from build123d import *

# Parameters (mm, degrees)
CROQUIS1_W              = 12
CROQUIS1_H              = 10
CROQUIS1_R              = 0.5
SALIENTE_EXTRUIR1_DEPTH = 0.7
CROQUIS2_R              = 1.5
SALIENTE_EXTRUIR2_DEPTH = 8.3
SALIENTE_EXTRUIR3_DEPTH = 0.7
SALIENTE_EXTRUIR4_DEPTH = 0.7
CORTAR_EXTRUIR1_REACH   = 13.916
CROQUIS5_R              = 1.5
REDONDEO1_R             = 0.5


with BuildPart() as part:
    # Croquis1 → Saliente-Extruir1 (new body)
    with BuildSketch(Plane(origin=(0, 0, 0), x_dir=(1, 0, 0), z_dir=(0, 1, 0))):
        Rectangle(CROQUIS1_W, CROQUIS1_H)
        with Locations(Location((0, 0, 0), (0, 0, 270))):
            Circle(CROQUIS1_R, mode=Mode.SUBTRACT)
    extrude(amount=SALIENTE_EXTRUIR1_DEPTH)

    # Croquis2 → Saliente-Extruir2 (add)
    with BuildSketch(Plane(origin=(0, 0.7, 0), x_dir=(1, 0, 0), z_dir=(0, 1, 0))):
        with Locations(Location((4, 3, 0), (0, 0, 90))):
            Circle(CROQUIS2_R)
        with Locations(Location((-4, -3, 0), (0, 0, 90))):
            Circle(CROQUIS2_R)
    extrude(amount=SALIENTE_EXTRUIR2_DEPTH)

    # Croquis3 → Saliente-Extruir3 (add)
    with BuildSketch(Plane(origin=(0, 3.3, 0), x_dir=(1, 0, 0), z_dir=(0, 1, 0))):
        Polygon((6, -0.6), (1.6, -0.6), (1.6, -5), (-6, -5), (-6, 5), (6, 5), align=None)
    extrude(amount=SALIENTE_EXTRUIR3_DEPTH)

    # Croquis4 → Saliente-Extruir4 (add)
    with BuildSketch(Plane(origin=(0, 8.3, 0), x_dir=(1, 0, 0), z_dir=(0, 1, 0))):
        Polygon((6, -0.6), (6, -5), (1.6, -5), (-6, -5), (-6, 5), (6, 5), align=None)
    extrude(amount=SALIENTE_EXTRUIR4_DEPTH)

    # Cortar-Extruir1: up to this face of the body (flat: up to its plane)
    cortar_extruir1_end = Plane(part.part.faces().sort_by_distance((-0.850469255, 3.3, -0.626661556))[0])
    # Croquis5 → Cortar-Extruir1 (cut, up to the picked face)
    with BuildSketch(Plane(origin=(0, 9, 0), x_dir=(1, 0, 0), z_dir=(0, 1, 0)), mode=Mode.PRIVATE) as cortar_extruir1_sk1:
        with Locations(Location((0, 0, 0), (0, 0, 270))):
            Circle(CROQUIS5_R)
    cortar_extruir1_tool1 = split(extrude(cortar_extruir1_sk1.sketch, amount=-CORTAR_EXTRUIR1_REACH, mode=Mode.PRIVATE), bisect_by=cortar_extruir1_end, keep=Keep.BOTH, mode=Mode.PRIVATE)
    add(cortar_extruir1_tool1.solids().sort_by(Axis((0, 9, 0), (0, -1, 0)))[0], mode=Mode.SUBTRACT)

    # Redondeo1
    redondeo1_edges = [part.edges().sort_by_distance(p)[0] for p in [
        (6, 3.65, -5),
        (-6, 3.65, -5),
        (-6, 3.65, 5),
        (1.6, 3.65, 5),
        (6, 3.65, 0.6),
        (6, 8.65, -5),
        (-6, 8.65, -5),
        (6, 8.65, 5),
        (6, 0.35, 5),
        (-6, 0.35, 5),
        (-6, 0.35, -5),
        (6, 0.35, -5),
    ]]
    fillet(redondeo1_edges, radius=REDONDEO1_R)


solid = part.part
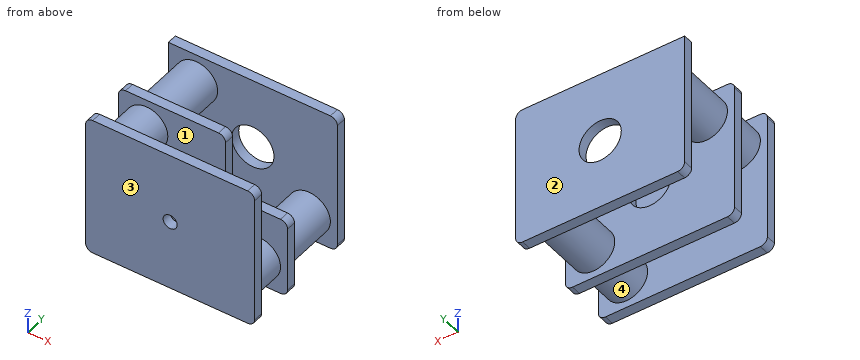
Model file for the job. Use its own axes, mm. Face numbers are marked on the shaded views. Give positions to 0.01 mm unless a question says otherwise; leave off trailing zeros. Order: outer loops, then holes, each group sorted by start corner. A loop starts at its lowest first (then second) coordinate and runs counter-clockwise, first axis right, second up. Notation, with made-up numbers: (5, 2) - (21, 2) arc R25 ccw to (21, 17) - close; hole circle Ø6 at (-27, -22.75). An arc over 180 degrees is marked (long way). Write item = value, one per line. Start each with the question number.
1. Cut at B-B, the plane z = 3. List the corners of the cut face in (x, y).
2. Cut at C-C, the plane x = 2. List the corners of the cut face in (y, z).
3. Two-plate mould, pull along Y, no slides. Class the marked faces 1, 2, 3 and 4: pulls with the +Y half, pulls with the -Y half, needs draft (parallel to the pull), parting line crosses it, or undercut.
4. Probe line 1 along Y through (x, z) = (2.75, -1); line 2 along X through (y, z) = (0.25, 0); line 3 along Y through (x, z) = (4.75, 4.75). List the from-to ranges inside material, lowest first.
5. Drop flat-ended pins along their axis: P1, Ø0.6, axis at x = 4, y = 4, coming from the +Z side; P2, Ø3.5, axis at x = 0, z = 0, coming from the -Y side; P3, Ø1.5, axis at x = -4, y = 5, coming from the -Z side. Give the stop position or say it passes through.
6. Cut at D-D, the plane y = 8. List the corners of the cut face in (x, z).
7. Cut at A-A, the plane x = 0. List the corners of the cut face in (y, z).
Taken from the geometry:
q1.outline = (-6, 0) - (6, 0) - (6, 0.7) - (-2.5, 0.7) - (-2.5, 3.3) - (1.6, 3.3) - (1.6, 4) - (-2.5, 4) - (-2.5, 8.3) - (6, 8.3) - (6, 9) - (-6, 9) - (-6, 8.3) - (-5.5, 8.3) - (-5.5, 4) - (-6, 4) - (-6, 3.3) - (-5.5, 3.3) - (-5.5, 0.7) - (-6, 0.7) - close
q2.outline = (0, -5) - (0.7, -5) - (0.7, 5) - (0, 5) - close; (3.3, -5) - (4, -5) - (4, 0.6) - (3.3, 0.6) - close; (8.3, -5) - (9, -5) - (9, 5) - (8.3, 5) - close
q3.face_1 = undercut
q3.face_2 = pulls with the +Y half
q3.face_3 = pulls with the -Y half
q3.face_4 = undercut
q4.line_1 = 0 to 0.7, 3.3 to 4, 8.3 to 9
q4.line_2 = -6 to -0.5, 0.5 to 6
q4.line_3 = 0 to 0.7, 8.3 to 9
q5.P1 = 0.6
q5.P2 = 0
q5.P3 = 1.5
q6.outline = circle Ø3 at (-4, 3); circle Ø3 at (4, -3)
q7.outline = (0, -5) - (0.7, -5) - (0.7, -0.5) - (0, -0.5) - close; (0, 0.5) - (0.7, 0.5) - (0.7, 5) - (0, 5) - close; (3.3, -5) - (4, -5) - (4, -1.5) - (3.3, -1.5) - close; (3.3, 1.5) - (4, 1.5) - (4, 5) - (3.3, 5) - close; (8.3, -5) - (9, -5) - (9, -1.5) - (8.3, -1.5) - close; (8.3, 1.5) - (9, 1.5) - (9, 5) - (8.3, 5) - close
